```python
from build123d import *

# Parameters (mm, degrees)
SKICA1_R                 = 1.5
P_IDAT_VYSUNUT_M1_DEPTH  = 23
SKICA2_OUTSIDE_W         = 17.264
SKICA2_OUTSIDE_H         = 30.264
ODEBRAT_VYSUNUT_M2_DEPTH = 26.079872408
SKICA3_R                 = 1.5
ODEBRAT_VYSUNUT_M3_DEPTH = 26.396850254
ODEBRAT_VYSUNUT_M4_DEPTH = 23.203603329


with BuildPart() as part:
    # Skica1 → Přidat vysunutím1 (new body)
    with BuildSketch(Plane(origin=(0, 0, 0), x_dir=(1, 0, 0), z_dir=(0, 1, 0))):
        with BuildLine():
            Line((-4, 0), (-4, 6))
            Line((-4, 6), (4, 6))
            Line((4, 6), (4, 0))
            ThreePointArc((4, 0), (0, -4), (-4, 0))
        make_face()
        with Locations(Location((0, 0, 0), (0, 0, 270))):
            Circle(SKICA1_R, mode=Mode.SUBTRACT)
    extrude(amount=P_IDAT_VYSUNUT_M1_DEPTH)

    # Skica2 outside → Odebrat vysunutím2 (cut, through all)
    with BuildSketch(Plane.ZY.offset(4)):
        with Locations((-1, 11.5)):
            Rectangle(SKICA2_OUTSIDE_W, SKICA2_OUTSIDE_H)
        with BuildLine():
            Line((-3, 23), (-3, 10))
            ThreePointArc((-3, 10), (-1.535533906, 6.464466094), (2, 5))
            Line((2, 5), (4, 5))
            Line((4, 5), (4, 0))
            Line((4, 0), (-6, 0))
            Line((-6, 0), (-6, 23))
            Line((-6, 23), (-3, 23))
        make_face(mode=Mode.SUBTRACT)
    extrude(amount=-ODEBRAT_VYSUNUT_M2_DEPTH, mode=Mode.SUBTRACT)

    # Skica3 → Odebrat vysunutím3 (cut, through all)
    with BuildSketch(Plane(origin=(0, 0, -6), x_dir=(-1, 0, 0), z_dir=(0, 0, -1))):
        with Locations((0, 19)):
            Circle(SKICA3_R)
        with BuildLine():
            Line((-4, 19), (-7.602186301, 24.874773566))
            Line((-7.602186301, 24.874773566), (9.845338693, 23.958039202))
            Line((9.845338693, 23.958039202), (4, 19))
            ThreePointArc((4, 19), (0, 23), (-4, 19))
        make_face()
    extrude(amount=-ODEBRAT_VYSUNUT_M3_DEPTH, mode=Mode.SUBTRACT)

    # Skica6 → Odebrat vysunutím4 (cut, through all)
    with BuildSketch(Plane.XZ.offset(-2)):
        Polygon((1.58771324, 2.75), (-1.58771324, 2.75), (-3.175426481, 0), (-1.58771324, -2.75), (1.58771324, -2.75), (3.175426481, 0), align=None)
    extrude(amount=-ODEBRAT_VYSUNUT_M4_DEPTH, mode=Mode.SUBTRACT)


solid = part.part
```
Input: part model. Units: mm. Frame: model coordinates. A direction names the side the tool comes from. Give positions to 0.01 mm unless a question says otherwise; leave off trailing zeros. Order: outer loops, then holes, each group sorted by start corner. A loop starts at its lowest first (then second) coordinate and runs counter-clockwise, first axis right, second up. Notation, with made-up numbers: M 28,21 L 47,21 A29 cw 47,60 Z; hole C 13.5,-35.5 d10. An arc over 180 degrees is marked long. One line per question, with ' | ' between items. Start each with the question number.
1. Pull-direction query (X, two-part tool) for faces 1 (the face through (0, 11, -6)), 2 (the face through (-2.39, 4.46, -1.36)), 3 (the face through (0, 3, 4)); classes: released by +X, released by -X, zero draft, split by the parting line, or undercut.
2. Section query B-B (x = 0). Return the cut outline in (y, z), and give its area (3 significant figures).
3. Section query A-A (y = 4.75). Return the cut outline in (x, z), and give its area (3 significant figures).
4. Material intervals for probe 1 along X at (y, z) = (1, 0); probe 2 along Y at (x, z) = (0, -5); probe 3 along Z at (x, y) = (0, 1.55), sorted ascending. Write a range as [from, to].
5. Access query for faces 4 (the face through (0, 5, 3)), 5 (the face through (1.4, 2, 1.3)), 6 (the face through (4, 7, -4)). Directions: +Z, -Z, +X, -X, +Y, -Y. A direction counts if a zero-diameter tool reaches every point of the face in a straight line with its end or side. Return the directions, or none.
6. Section query C-C (z = -0.25). Return the cut outline in (x, y).
7. Section query D-D (y = 7.5). Return the cut outline in (x, z).
8. First-contact query: pin 1 Ø2.5 at (x, z) = (0, 0) entering from +Y; pin 2 Ø1 at (x, y) = (-1.5, 18) entering from +Z; pin 3 Ø3 at (x, z) = (1, 0) entering from +Y; pin 4 Ø1.6 at (x, z) = (0, 3) entering from +Y. Flat tips, straight axial feed; report the tip coordinate or a pass-through.
Here are the results:
1) face 1: zero draft | face 2: undercut | face 3: split by the parting line
2) outline: M 0,-6 L 17.5,-6 L 17.5,-3 L 10,-3 A5 cw 8.44,-2.75 L 2,-2.75 L 2,-1.5 L 0,-1.5 Z; M 0,1.5 L 2,1.5 L 2,2.75 L 5,2.75 L 5,4 L 0,4 Z; M 20.5,-6 L 23,-6 L 23,-3 L 20.5,-3 Z | area: 73.5 mm²
3) outline: M -4,-6 L 4,-6 L 4,0 A4 ccw -4,0 Z; hole M -3.18,0 L -1.59,-2.75 L 1.59,-2.75 L 3.18,0 L 1.59,2.75 L -1.59,2.75 Z | area: 46.9 mm²
4) probe 1: [-4, -1.5], [1.5, 4] | probe 2: [0, 17.5], [20.5, 23] | probe 3: [-6, -1.5], [1.5, 4]
5) face 4: +Z, +X, -X, +Y | face 5: +Y | face 6: +Z, -Z, +X, +Y, -Y
6) outline: M -4,0 L -1.48,0 L -1.48,2 L -3.03,2 L -3.03,5.53 L -4,5.53 Z; M 1.48,0 L 4,0 L 4,5.53 L 3.03,5.53 L 3.03,2 L 1.48,2 Z
7) outline: M -4,-6 L 4,-6 L 4,-2.33 L 1.83,-2.33 L 1.59,-2.75 L -1.59,-2.75 L -1.83,-2.33 L -4,-2.33 Z
8) pin 1: through | pin 2: z = -3 | pin 3: y = 2 | pin 4: y = 5
